from build123d import *

# Parameters (mm, degrees)
F0_W     = 15.2
F0_H     = 15.2
F0_W_2   = 30
F0_H_2   = 4
F0_W_3   = 4
F0_H_3   = 30
F1_DEPTH = 4
F2_DEPTH = 36
F3_DEPTH = 15.2
F4_R     = 3.99999
F6_R     = 1.99999


# Not quite as in the source:
# - a fillet or chamfer is up to 0.001 mm smaller than in the source, because OpenCascade refuses the exact size
# - a feature of the source that left no trace in its solid (it failed there, or was rolled back) is left out


with BuildPart() as f1:
    # F0 (on Top) → F1 (new body)
    with BuildSketch(Plane.XY):
        Polygon((-4, 15.2), (-4, -4), (19.2, -4), (19.2, 19.2), (0, 19.2), (-4, 19.2), align=None)
        with Locations((7.6, 7.6)):
            Rectangle(F0_W, F0_H, mode=Mode.SUBTRACT)
        with Locations((-19, 17.2)):
            Rectangle(F0_W_2, F0_H_2)
        with Locations((-2, 34.2)):
            Rectangle(F0_W_3, F0_H_3)
        with Locations((7.6, 7.6)):
            Rectangle(F0_W, F0_H)
    extrude(amount=F1_DEPTH)

    # F0 (on Top) → F2 (join)
    with BuildSketch(Plane.XY):
        Polygon((-4, 15.2), (-4, -4), (19.2, -4), (19.2, 19.2), (0, 19.2), (-4, 19.2), align=None)
        with Locations((7.6, 7.6)):
            Rectangle(F0_W, F0_H, mode=Mode.SUBTRACT)
    extrude(amount=F2_DEPTH)

    # F0 (on Top) → F3 (join)
    with BuildSketch(Plane.XY):
        with Locations((-19, 17.2)):
            Rectangle(F0_W_2, F0_H_2)
        with Locations((-2, 34.2)):
            Rectangle(F0_W_3, F0_H_3)
    extrude(amount=F3_DEPTH)

    # F4 (radius 4 in the source; OpenCascade refuses exactly that, so slightly less here)
    f4_edges = [f1.edges().sort_by_distance(p)[0] for p in [
        (-4, -4, 18),
        (19.2, -4, 18),
        (19.2, 19.2, 18),
        (-4, 19.2, 7.6),
        (-4, 19.2, 25.6),
    ]]
    fillet(f4_edges, radius=F4_R)

    # F6 (radius 2 in the source; OpenCascade refuses exactly that, so slightly less here)
    f6_edges = [f1.edges().sort_by_distance(p)[0] for p in [
        (0, 49.2, 7.6),
        (-4, 49.2, 7.6),
        (-34, 19.2, 7.6),
        (-34, 15.2, 7.6),
    ]]
    fillet(f6_edges, radius=F6_R)


solid = f1.part
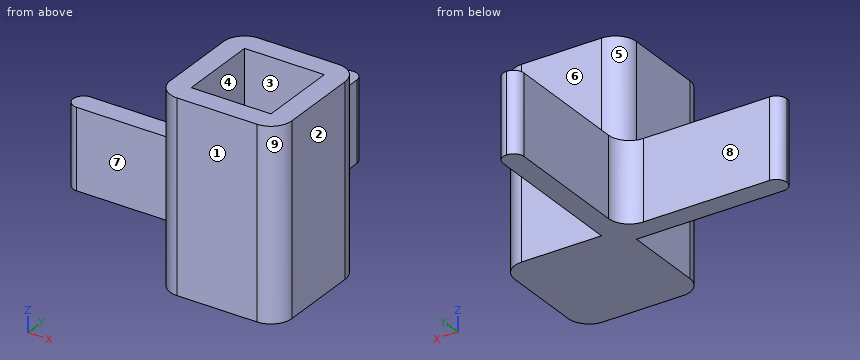
Design review of the part built by this model. Coordinates are the model's own, in mm. Face numbers are marked on the shaded views. A direction names the side the tool comes from. Coordinates: 2 decimals unless noted, no trailing zeros. Loops run counter-clockwise (first coordinate to the right, second up) from the corner with the lowest first, then second, coordinate; pieces in that order, holes last. Notation, with made-up numbers: (85, 13.25) -> (131, 13.25) arc R20 cw to (131, 19.25) -> close; hole circle Ø4 at (28.25, -18.75). An arc over 180 degrees is marked (long way). Use a Markdown table: item, result. Add a question column.
Item 1: Wall thickness on L1, parallel to Y at x = 2.5, z = 15.5; L2, parallel to X at y = 44, z = 4: over which ranges is each line inside the solid? List them lowest first. Write a range as from..to.
Item 2: Clearance check with flat-ended pins moving along their axes: P1, Ø4, axis at y = 6, z = 27.5, coming from the -X side; P2, Ø12, axis at y = 10.5, z = 12, coming from the -X side; P3, Ø4.5, axis at x = -13.5, z = 8, coming from the -Y side. State where each tip first meets the part, or that it passes through.
Item 3: We need section C-C, the plane x = 3. Write out the cut boundary in (y, z).
Item 4: The part is to be moulded in two halves that separate along Y. For the marked faces 1, 2, 3 and 4, say which applies: +Y half, -Y half, draft (parallel to the pull), parting line (faces both ways), or undercut.
Item 5: Machinability: for the marked faces 5, 6, 7, 8 and 9, which of the approach directions +Z, -Z, +X, -X, +Y, -Y give a long, thin tool a straight path to every point of the face, cutting with its end or side? Answer none if there is none.
Item 6: We need section A-A, the plane z = 28.5. Write out the cut boundary in (x, y), and give its area (3 significant figures).
Numbers:
| question | item | result |
|---|---|---|
| 1 | L1 | y = -4..0, 15.2..19.2 |
| 1 | L2 | x = -4..0 |
| 2 | P1 | stops at x = -4 |
| 2 | P2 | stops at x = -33.87 |
| 2 | P3 | stops at y = 15.2 |
| 3 | outline | (-4, 0) -> (19.2, 0) -> (19.2, 36) -> (15.2, 36) -> (15.2, 4) -> (0, 4) -> (0, 36) -> (-4, 36) -> close |
| 4 | face 1 | -Y half |
| 4 | face 2 | draft |
| 4 | face 3 | undercut |
| 4 | face 4 | undercut |
| 5 | face 5 | +Z, -X, +Y |
| 5 | face 6 | +Z, -Z, +X, +Y |
| 5 | face 7 | +Z, -Z, -X, -Y |
| 5 | face 8 | +Z, -Z, -X, +Y |
| 5 | face 9 | +Z, -Z, +X, -Y |
| 6 | outline | (-4, 0) arc R4 ccw to (0, -4) -> (15.2, -4) arc R4 ccw to (19.2, 0) -> (19.2, 15.2) arc R4 ccw to (15.2, 19.2) -> (0, 19.2) arc R4 ccw to (-4, 15.2) -> close; hole (0, 0) -> (15.2, 0) -> (15.2, 15.2) -> (0, 15.2) -> close |
| 6 | area | 293 mm^2 |
